Geometry check sheet. Reference: the model listing, model coordinates, mm. A direction names the side the tool comes from. Round coordinates to 2 decimals unless told otherwise and drop trailing zeros. Order: outer loops, then holes, each group sorted by start corner. A loop starts at its lowest first (then second) coordinate and runs counter-clockwise, first axis right, second up.
(1) Cross-section at A-A on y = -10. Enter the section's corners in (x, z), and give its area (3 significant figures).
(2) Thickness scan on L1, parallel to Y at x = -0.5, z = -4; L2, parallel to X at y = 4, z = -1.5; L3, parallel to Z at x = 0.75, y = 3.5. Record the ranges inside material, lowest first.
(3) Gauge pin test, flat ends, axial feed: P1, Ø3, axis at y = -4.5, z = -1, coming from the -X side; P2, Ø5, axis at x = 0.5, y = -9, coming from the -Z side; P3, Ø2, axis at y = -15.5, z = -1.5, coming from the +X side. Record the tip position at first contact, or that the pin passes through.
(4) Set-up check for faces 4 (the face through (-2.155, 4.521, -1.267)), 5 (the face through (0.9, -14.49, 2.86)), 6 (the face through (0, -30, 0)): record each of +Z, -Z, +X, -X, +Y, -Y from which the full face is reachable in a straight line by a thin tool's end or side.
(5) Cross-section at B-B on y = 2.5. Enter the section's corners in (x, z).
(6) Draft check along X on faces 1 (the face through (0, 3, -5)), 2 (the face through (0, 5, 2.5)), 3 (the face through (3.3, 0, 0.1)). Enter one of: pulls with the +X half, pulls with the -X half, needs draft (parallel to the pull), parting line crosses it, or undercut.
from build123d import *

# Parameters (mm, degrees)
ESQUISSE2_R             = 3
BASE_EXTRUSION_DEPTH    = 30
CHANFREIN1_SIZE         = 0.6
ENL_V_MAT_EXTRU_1_DEPTH = 3


with BuildPart() as part:
    # Esquisse2 → Base-Extrusion (new body)
    with BuildSketch(Plane(origin=(0, 0, 0), x_dir=(1, 0, 0), z_dir=(0, 1, 0))):
        with Locations(Location((0, 0, 0), (0, 0, 270))):  # turned: the seam where the file's is
            Circle(ESQUISSE2_R)
    extrude(amount=-BASE_EXTRUSION_DEPTH)

    # Chanfrein1
    chanfrein1_edges = [part.edges().sort_by_distance(p)[0] for p in [
        (0, -30, -3),
    ]]
    chamfer(chanfrein1_edges, length=CHANFREIN1_SIZE)

    # Esquisse5 → Boss.-Révol.1 (revolve)
    with BuildSketch(Plane.XY, mode=Mode.PRIVATE) as boss_r_vol_1_sk:
        with BuildLine():
            Line((2.5, 6), (2.5, 3))
            Line((2.5, 3), (0, 1.556624327))
            Line((0, 1.556624327), (0, 0))
            Line((0, 0), (5, 0))
            Line((5, 0), (5, 5.4))
            ThreePointArc((5, 5.4), (4.824264069, 5.824264069), (4.4, 6))
            Line((4.4, 6), (2.5, 6))
        make_face()
    revolve(boss_r_vol_1_sk.sketch.rotate(Axis((0, 6, 0), (0, -1, 0)), 90), axis=Axis((0, 6, 0), (0, -1, 0)))  # turned: the seam where the file's is

    # Esquisse7 → Enlèv. mat.-Extru.1 (cut)
    with BuildSketch(Plane(origin=(0, 6, 0), x_dir=(-1, 0, 0), z_dir=(0, 1, 0))):
        Polygon((1.443375673, 2.5), (-1.443375673, 2.5), (-2.886751346, 0), (-1.443375673, -2.5), (1.443375673, -2.5), (2.886751346, 0), align=None)
    extrude(amount=-ENL_V_MAT_EXTRU_1_DEPTH, mode=Mode.SUBTRACT)


solid = part.part
Found:
1. outline: circle Ø6 at (0, 0)
1. area: 28.3 mm2
2. L1: y = 0 to 6
2. L2: x = -4.77 to -2.02, 2.02 to 4.77
2. L3: z = -4.94 to -2.5, 2.5 to 4.94
3. P1: stops at x = -3
3. P2: stops at z = -3
3. P3: stops at x = 2.96
4. face 4: +Y
4. face 5: -Y
4. face 6: +Z, -Z, +X, -X, -Y
5. outline: circle Ø10 at (0, 0); hole circle Ø3.27 at (0, 0)
6. face 1: parting line crosses it
6. face 2: undercut
6. face 3: needs draft
